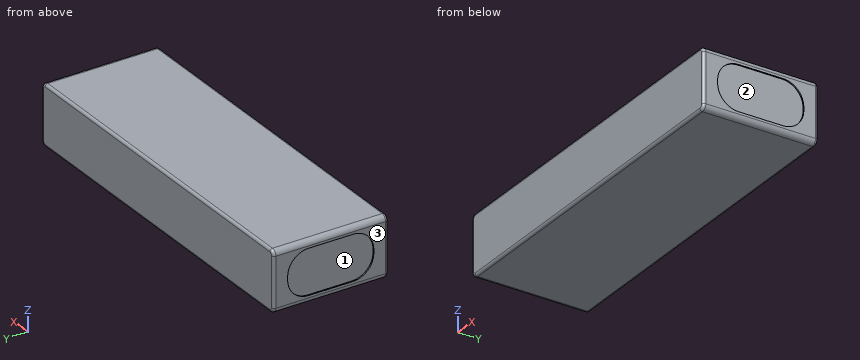
from build123d import *

# Parameters (mm, degrees)
SKETCH1_W           = 135
SKETCH1_H           = 44
BOSS_EXTRUDE1_DEPTH = 23
CUT_EXTRUDE1_DEPTH  = 0.5
CUT_EXTRUDE2_DEPTH  = 0.5
FILLET1_R           = 2
FILLET2_R           = 1


with BuildPart() as part:
    # Sketch1 → Boss-Extrude1 (new body)
    with BuildSketch(Plane(origin=(0, 0, -15), x_dir=(-1, 0, 0), z_dir=(0, 0, -1))):
        with Locations((-1.5, 0)):
            Rectangle(SKETCH1_W, SKETCH1_H)
    extrude(amount=-BOSS_EXTRUDE1_DEPTH)

    # Sketch2 → Cut-Extrude1 (cut)
    with BuildSketch(Plane(origin=(69, 0, 0), x_dir=(0, 0, -1), z_dir=(1, 0, 0))):
        with BuildLine():
            Line((-5.125, 8.5), (-5.125, -8.5))
            ThreePointArc((-5.125, -8.5), (-2.781854249, -14.156854249), (2.875, -16.5))
            Line((2.875, -16.5), (4.125, -16.5))
            ThreePointArc((4.125, -16.5), (9.781854249, -14.156854249), (12.125, -8.5))
            Line((12.125, -8.5), (12.125, 8.5))
            ThreePointArc((12.125, 8.5), (9.781854249, 14.156854249), (4.125, 16.5))
            Line((4.125, 16.5), (2.875, 16.5))
            ThreePointArc((2.875, 16.5), (-2.781854249, 14.156854249), (-5.125, 8.5))
        make_face()
    extrude(amount=-CUT_EXTRUDE1_DEPTH, mode=Mode.SUBTRACT)

    # Sketch3 → Cut-Extrude2 (cut)
    with BuildSketch(Plane.ZY.offset(66)):
        with BuildLine():
            Line((-2.875, 16.5), (-4.125, 16.5))
            ThreePointArc((-4.125, 16.5), (-9.781854249, 14.156854249), (-12.125, 8.5))
            Line((-12.125, 8.5), (-12.125, -8.5))
            ThreePointArc((-12.125, -8.5), (-9.781854249, -14.156854249), (-4.125, -16.5))
            Line((-4.125, -16.5), (-2.875, -16.5))
            ThreePointArc((-2.875, -16.5), (2.781854249, -14.156854249), (5.125, -8.5))
            Line((5.125, -8.5), (5.125, 8.5))
            ThreePointArc((5.125, 8.5), (2.781854249, 14.156854249), (-2.875, 16.5))
        make_face()
    extrude(amount=-CUT_EXTRUDE2_DEPTH, mode=Mode.SUBTRACT)

    # Fillet1
    fillet1_edges = [part.edges().sort_by_distance(p)[0] for p in [
        (-66, 0, 8),
        (69, 0, 8),
        (-66, 0, -15),
        (69, 0, -15),
    ]]
    fillet(fillet1_edges, radius=FILLET1_R)

    # Fillet2
    fillet2_edges = [part.edges().sort_by_distance(p)[0] for p in [
        (1.5, -22, -15),
        (1.5, 22, -15),
        (-66, 22, -3.5),
        (1.5, 22, 8),
        (69, 22, -3.5),
        (68.414213562, 22, 7.414213562),
        (68.414213562, 22, -14.414213562),
        (-65.414213562, 22, 7.414213562),
        (-65.414213562, 22, -14.414213562),
        (-66, -22, -3.5),
        (69, -22, -3.5),
        (1.5, -22, 8),
        (68.414213562, -22, 7.414213562),
        (68.414213562, -22, -14.414213562),
        (-65.414213562, -22, 7.414213562),
        (-65.414213562, -22, -14.414213562),
    ]]
    fillet(fillet2_edges, radius=FILLET2_R)


solid = part.part
For this review, take the finished solid that the model builds, in its own axes (mm). Face numbers are marked on the shaded views. A direction names the side the tool comes from. Give positions to 0.01 mm unless a question says otherwise; leave off trailing zeros.
Item 1: Insertion check: pin 1 (0.6 mm diameter, centred on x = -66, y = -2.5, fed in from -Z); pin 2 (5 mm diameter, centred on y = 2, z = -5.5, fed in from +X); pin 3 (8.5 mm diameter, centred on y = -6.5, z = -4, fed in from -X); pin 4 (8 mm diameter, centred on y = -14.5, z = -0.5, fed in from +X). Each pin has a flat end and moves straight along its axis. Give the tip position at first contact, or say it passes through.
Item 2: Tool access review of the marked faces 1, 2 and 3: name each direction out of +Z, -Z, +X, -X, +Y, -Y from which nothing blocks a thin tool from reaching the whole face with its end or side.
Item 3: For line 1 along X through (y, z) = (-6, -10); line 2 along X through (y, z) = (19.5, 6.5), list the stretches that pass through material, from the lowest coordinate up.
Calculated:
1. pin 1: stops at z = -14.05
1. pin 2: stops at x = 68.5
1. pin 3: stops at x = -65.5
1. pin 4: stops at x = 69
2. face 1: -X
2. face 2: +X
2. face 3: +Z, -Z, -X, +Y, -Y
3. line 1: x = -65.5 to 68.5
3. line 2: x = -65.94 to 68.94
